Autodesk Inventor part; units mm, degrees
ref_plane "Work Plane1" through (20, 11, 20) normal (0, 1, 0) x (1, 0, 0)
ref_plane "Work Plane2" through (10, 10, 0) normal (0, -1, 0) x (1, 0, 0)
ref_plane "YZ Plane" through (0, 0, 0) normal (1, 0, 0) x (0, 1, 0)
sketch "Sketch1" plane through (0, 0, 0) normal (0, 0, 1) x (1, 0, 0)
  line L0 (0, 0) -> (20, 0)
  line L1 (20, 0) -> (20, 14)
  line L2 (20, 14) -> (0, 14)
  line L3 (0, 14) -> (0, 0)
  circle A0 centre (10, 14) radius 4
  line L4 (7.9329, 10) -> (16.1844, 10) construction
  line L5 (6, 14) -> (0, 14)
  line L6 (14, 14) -> (20, 14)
  line L7 (20, 14) -> (0, 14)
  line L8 (0, 14) -> (0, 22)
  line L9 (0, 22) -> (20, 22)
  line L10 (20, 22) -> (20, 14)
  line L11 (20, 13.5) -> (13.9686, 13.5)
  line L12 (13.9686, 13.5) -> (13.9686, 14.5)
  line L13 (13.9686, 14.5) -> (20, 14.5)
  line L14 (20, 14.5) -> (20, 13.5)
  point P0 (20, 7)
  point P1 (0, 7)
  point P2 (17, 14)
  point P3 (3, 14)
  point P4 (13.9686, 14)
  point P5 (0, 14)
  dimension "d0" = 8
  dimension "d1" = 10
  dimension "d2" = 20
  dimension "d5" = 8
  dimension "d6" = 1
extrude "Extrusion1" add sketch "Sketch1" along normal blind 20 contours L3 L2 A0 L11 L1 L0 | L8 L9 L10 L13 A0 L2 | L11 A0 L2 L1
chamfer "Chamfer1" distance 1 angle 45 2 edges at (6.0079, 13.7495, 0) (6.0079, 13.7495, 20)
ref_plane "Work Plane1" through (20, 11, 20) normal (0, 1, 0) x (1, 0, 0)
sketch "Sketch2" plane through (0, 22, 0) normal (0, 1, 0) x (1, 0, 0)
  line L0 (15, -20) -> (14, -19)
  line L1 (20, -20) -> (15, -20)
  line L2 (20, 0) -> (20, -20)
  line L3 (20, 0) -> (15, 0)
  line L4 (14, -1) -> (15, 0)
  line L5 (14, -1) -> (14, -19)
  line L6 (14, -15.8523) -> (20, -15.8523)
  line L7 (15.4123, -7.25) -> (18.5877, -7.25)
  line L8 (18.5877, -7.25) -> (20.1754, -10) construction
  line L9 (20.1754, -10) -> (18.5877, -12.75) construction
  line L10 (18.5877, -12.75) -> (15.4123, -12.75)
  line L11 (15.4123, -12.75) -> (13.8246, -10)
  line L12 (13.8246, -10) -> (15.4123, -7.25)
  line L13 (18.5877, -12.75) -> (22.4339, -12.75)
  line L14 (22.4339, -12.75) -> (22.4339, -7.25)
  line L15 (22.4339, -7.25) -> (18.5877, -7.25)
  line L16 (18.5877, -7.25) -> (18.5877, -12.75) construction
  point P0 (0, 0)
  point P1 (17, -10)
  point P2 (20, -10)
  point P3 (17, -15.8523)
  point P4 (17, -10)
  dimension "d10" = 5.5
extrude "Extrusion2" cut sketch "Sketch2" against normal blind 3 from surface at -11 contours L11 L12 L5 | L5 L12 L7 L15 L2 L13 L10 L11 | L2 L15 L14 L13
hole "Hole1" at (17, 22, 10) direction (0, -1, 0) diameter 3.2 end through all counterbore diameter 6.2 counterbore depth 3.58
chamfer "Chamfer2" distance 5 angle 45 2 edges at (20, 20.21, 9.219) (20, 20.21, 10.781)
ref_plane "Work Plane2" through (10, 10, 0) normal (0, -1, 0) x (1, 0, 0)
sketch "Sketch3" plane through (10, 10, 0) normal (0, -1, 0) x (1, 0, 0)
  line L0 (-5, 0) -> (5, 0)
  line L1 (5, 20) -> (-5, 20)
  line L2 (-10, 20) -> (10, 20)
  line L3 (0, 20) -> (0, 0)
  circle A0 centre (0, 14) radius 3.05
  circle A1 centre (0, 6) radius 3.05
  point P0 (-10, 0)
  point P1 (4.9749, 0)
  point P2 (4.9749, 20)
  dimension "d24" = 6.1
  dimension "d25" = 6.1
  dimension "d26" = 6
  dimension "d27" = 6
extrude "Extrusion3" cut sketch "Sketch3" along normal blind 7 and the other way blind 2
hole "Hole2" at (10, 10, 6) at (10, 10, 14) direction (0, -1, 0) diameter 3.2 end through all
equation "\"d27\" = d26"
properties part number "Y Rod Holder"
Input: part model. Units: mm. Frame: model coordinates. A direction names the side the tool comes from. Coordinates: 2 decimals unless noted, no trailing zeros. Order: outer loops, then holes, each group sorted by start corner. A loop starts at its lowest first (then second) coordinate and runs counter-clockwise, first axis right, second up.
1. Cut plane A-A, the plane x = 10. Return loops of the section in (y, z).
Checked values:
outline: (0, 0) - (9, 0) - (10, 1) - (10, 2.95) - (3, 2.95) - (3, 4.4) - (0, 4.4) - close; (0, 7.6) - (3, 7.6) - (3, 9.05) - (10, 9.05) - (10, 10.95) - (3, 10.95) - (3, 12.4) - (0, 12.4) - close; (0, 15.6) - (3, 15.6) - (3, 17.05) - (10, 17.05) - (10, 19) - (9, 20) - (0, 20) - close; (18, 1) - (19, 0) - (22, 0) - (22, 20) - (19, 20) - (18, 19) - close
2. Access query for faces 1 (the flat face through (18, 10, 7.25)), 2 (the flat face through (15, 14.5, 10)), 3 (the cylindrical face through (10.97, 1.48, 12.73)). Directions: +Z, -Z, +X, -X, +Y, -Y. A direction counts if a zero-diameter tool reaches every point of the face in a straight line with its end or side. Return the directions, or none.
Checked values:
face 1: +X
face 2: +Z, -Z, +X
face 3: -Y
3. Contact query for a flat-ended pin moving along its axis: P1, Ø5, axis at x = 17, z = 10, coming from the +Y side. Output: stop coordinate, or through.
Checked values:
P1: stops at y = 18.42
4. Cut plane B-B, the plane z = 1.75. Return loops of the section in (x, y).
Checked values:
outline: (0, 0) - (20, 0) - (20, 14) - (14, 14) arc R4 cw (long way) to (13.97, 14.5) - (20, 14.5) - (20, 22) - (0, 22) - close
5. Draft query along Z for faces 4 (the cylindrical face through (12.91, 7.15, 14.92)), 5 (the conical face through (5.845, 13.611, 0.826)), 6 (the flat face through (18.2, 8, 8.7)), 7 (the flat face through (10, 0, 10)). Return one class per face: +Z half, -Z half, draft (parallel to the pull), parting line (faces both ways), or undercut.
Checked values:
face 4: undercut
face 5: -Z half
face 6: undercut
face 7: draft
6. Ray query, line 1 along Z through (x, y) = (10, 1.3); line 2 along Z through (x, y) = (9.25, 7.25); line 3 along Y through (x, z) = (16, 12.25). Return the intervals inside material, ascending.
Checked values:
line 1: z = 0 to 4.4, 7.6 to 12.4, 15.6 to 20
line 2: z = 0 to 3.04, 8.96 to 11.04, 16.96 to 20
line 3: y = 0 to 8, 11 to 14, 14.5 to 18.42
7. Cut plane C-C, the plane y = 2. Return loops of the section in (x, z), plus the area to 3 significant figures.
Checked values:
outline: (0, 0) - (20, 0) - (20, 20) - (0, 20) - close; hole circle Ø3.2 at (10, 6); hole circle Ø3.2 at (10, 14); hole circle Ø3.2 at (17, 10)
area: 376 mm2
8. Cut plane D-D, the plane z = 10.5. Return loops of the section in (x, y), plus the area to 3 significant figures.
Checked values:
outline: (0, 0) - (15.48, 0) - (15.48, 8) - (14.11, 8) - (14.11, 11) - (15.48, 11) - (15.48, 14) - (14, 14) arc R4 cw (long way) to (13.97, 14.5) - (15.48, 14.5) - (15.48, 18.42) - (13.94, 18.42) - (13.94, 22) - (0, 22) - close; (18.52, 0) - (20, 0) - (20, 8) - (18.52, 8) - close; (18.52, 11) - (20, 11) - (20, 14) - (18.52, 14) - close; (18.52, 14.5) - (20, 14.5) - (20, 18.42) - (18.52, 18.42) - close
area: 302 mm2
